Job drawing, mm, ordinate dimensions from the low corner. One solid piece. Round coordinates to 2 decimals unless told otherwise and drop trailing zeros. Loops run counter-clockwise (first coordinate to the right, second up) from the corner with the lowest first, then second, coordinate; pieces in that order, holes last. Notation, with made-up numbers: M -16.5,5.5 L 7.5,5.5 A14 cw 7.5,29.5 Z; hole C 76,48.5 d9. An arc over 180 degrees is marked long. Put each result on its own line as item: value. Start each with the question number.
1) Slice it at A-A on x = 35. Give the cut face in (y, z), then the cut area to 3 significant figures.
2) Pull direction Y, two halves, no side cores. Call the marked faces 1, 2 and 3: +Y half, -Y half, draft (parallel to the pull), parting line (faces both ways), or undercut.
3) Slice it at C-C on y = 14. Give the cut face in (x, z).
4) Slice it at B-B on z = 1.2. Give the cut face in (x, y).
5) Probe line 1 along Y through (x, z) = (5, 1.8); line 2 along X through (y, z) = (6.75, 0.45); line 3 along Y through (x, z) = (15.5, 1.9). List the from-to ranges inside material, lowest first.
6) Drop a flat-ended pin along its axis: pin 1 Ø1.9 at (x, y) = (15, 15) entering from +Z. Give the stop position or say it passes through.
7) Slice it at D-D on x = 15. Give the cut face in (y, z), then the cut area to 3 significant figures.
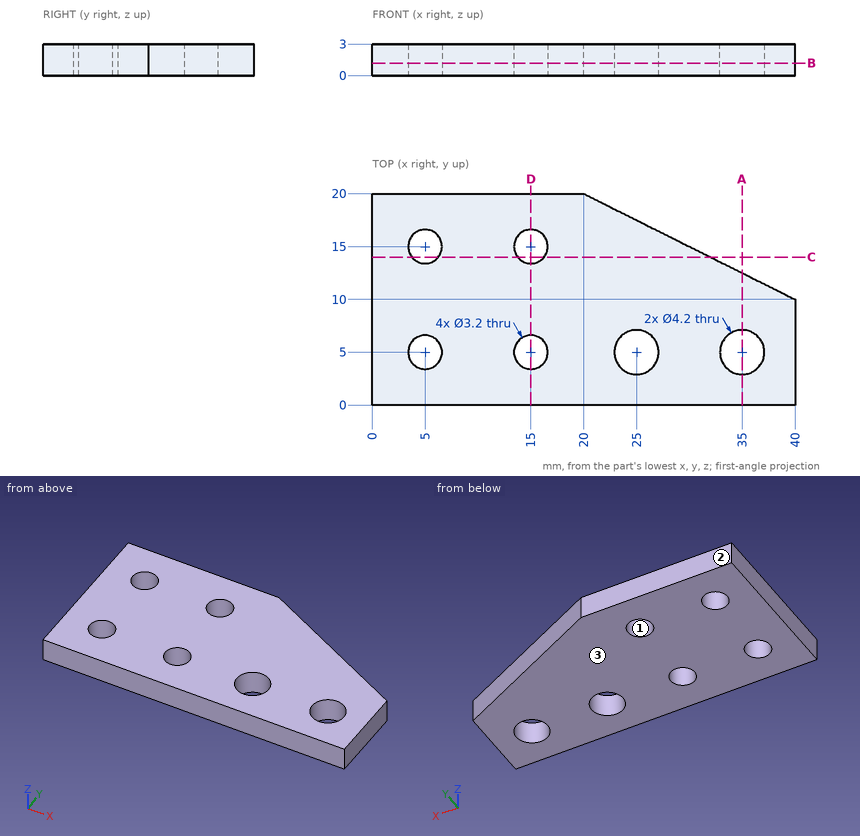
Recorded:
1. outline: M 0,0 L 2.9,0 L 2.9,3 L 0,3 Z; M 7.1,0 L 12.5,0 L 12.5,3 L 7.1,3 Z
1. area: 24.9 mm2
2. face 1: undercut
2. face 2: +Y half
2. face 3: draft
3. outline: M 0,0 L 3.75,0 L 3.75,3 L 0,3 Z; M 6.25,0 L 13.75,0 L 13.75,3 L 6.25,3 Z; M 16.25,0 L 32,0 L 32,3 L 16.25,3 Z
4. outline: M 0,0 L 40,0 L 40,10 L 20,20 L 0,20 Z; hole C 5,5 d3.2; hole C 5,15 d3.2; hole C 15,5 d3.2; hole C 15,15 d3.2; hole C 25,5 d4.2; hole C 35,5 d4.2
5. line 1: y = 0 to 3.4, 6.6 to 13.4, 16.6 to 20
5. line 2: x = 0 to 23.84, 26.16 to 33.84, 36.16 to 40
5. line 3: y = 0 to 3.48, 6.52 to 13.48, 16.52 to 20
6. pin 1: passes through
7. outline: M 0,0 L 3.4,0 L 3.4,3 L 0,3 Z; M 6.6,0 L 13.4,0 L 13.4,3 L 6.6,3 Z; M 16.6,0 L 20,0 L 20,3 L 16.6,3 Z
7. area: 40.8 mm2
